```python
from build123d import *

# Parameters (mm, degrees)
SKETCH2_W           = 8.2
SKETCH2_H           = 8.3
SKETCH2_R           = 0.833443519
SKETCH2_R_2         = 0.823803164
BOSS_EXTRUDE1_DEPTH = 1.35
SKETCH3_W           = 1.2
SKETCH3_H           = 3.1
BOSS_EXTRUDE2_DEPTH = 0.25


with BuildPart() as part:
    # Sketch2 → Boss-Extrude1 (new body, symmetric)
    with BuildSketch(Plane.XY):
        Rectangle(SKETCH2_W, SKETCH2_H)
        with Locations((-2, -2.55)):
            Circle(SKETCH2_R, mode=Mode.SUBTRACT)
        with Locations((2, -2.55)):
            Circle(SKETCH2_R_2, mode=Mode.SUBTRACT)
    extrude(amount=BOSS_EXTRUDE1_DEPTH, both=True)

    # Sketch3 → Boss-Extrude2 (add, symmetric)
    with BuildSketch(Plane.XY):
        with Locations((0, -5.7)):
            Rectangle(SKETCH3_W, SKETCH3_H)
        with Locations((2.5, -5.7)):
            Rectangle(SKETCH3_W, SKETCH3_H)
        with Locations((-2.5, -5.7)):
            Rectangle(SKETCH3_W, SKETCH3_H)
    extrude(amount=BOSS_EXTRUDE2_DEPTH, both=True)


solid = part.part
```
Geometry check sheet. Reference: the model listing, model coordinates, mm. A direction names the side the tool comes from. Give positions to 0.01 mm unless a question says otherwise; leave off trailing zeros. Loops run counter-clockwise (first coordinate to the right, second up) from the corner with the lowest first, then second, coordinate; pieces in that order, holes last. Notation, with made-up numbers: (80.5, 68) - (100.5, 68) arc R21 ccw to (100.5, 91) - close; hole circle Ø3 at (34, 10). An arc over 180 degrees is marked (long way). Use CSV: the item, a comma, the result in double quotes. Start each with the question number.
Q1. Scan lines: probe 1 along Y at (x, z) = (-2, 0.6); probe 2 along Y at (x, z) = (2, 0.15); probe 3 along X at (y, z) = (-2.75, -0.6). Record each from-to range of solid material in increasing order. Write a range as from..to.
Q2. Section check A-A, the plane y = -2.55. Record the cut outline in (x, z), and give its area (3 significant figures).
Q3. Section check D-D, the plane x = -3.5. Record the cut outline in (y, z), and give its area (3 significant figures).
Q4. Section check B-B, the plane z = -0.1. Record the cut outline in (x, y), and give its area (3 significant figures).
Q5. Go/stop test with flat-tipped pins: pin 1 Ø0.6 at (y, z) = (-5.5, 0) entering from -X; pin 2 Ø1.3 at (x, y) = (2.5, -6.5) entering from -Z; pin 3 Ø1.3 at (x, y) = (-2.5, -5.5) entering from +Z; pin 4 Ø1.5 at (x, y) = (2, -2.55) entering from +Z. Record where each tip stops, or that it passes through.
Q6. Release check for a two-part mould opening along Y. For faces 4 (the face through (1.346, -3.051, -0.019)), 5 (the face through (4.1, 0, 0)), 6 (the face through (0, 4.15, 0)), 7 (the face through (-2.833, -2.513, -0.019)) record: +Y half, -Y half, draft (parallel to the pull), parting line (faces both ways), or undercut.
Q7. Section check C-C, the plane x = -1.75. Record the cut outline in (y, z).
Q8. Access from +Z, -Z, +X, -X, +Y, -Y to the whole of each face (thin tool, end or side, straight path). Record for faces 1 (the face through (-4.1, 0, 0)), 2 (the face through (-2.5, -5.7, -0.25)), 3 (the face through (0, -6, 0.25)).
Findings below:
1,probe 1,"y = -4.15..-3.38, -1.72..4.15"
1,probe 2,"y = -7.25..-3.37, -1.73..4.15"
1,probe 3,"x = -4.1..-2.81, -1.19..1.2, 2.8..4.1"
2,outline,"(-4.1, -1.35) - (-2.83, -1.35) - (-2.83, 1.35) - (-4.1, 1.35) - close; (-1.17, -1.35) - (1.18, -1.35) - (1.18, 1.35) - (-1.17, 1.35) - close; (2.82, -1.35) - (4.1, -1.35) - (4.1, 1.35) - (2.82, 1.35) - close"
2,area,"13.2 mm^2"
3,outline,"(-4.15, -1.35) - (4.15, -1.35) - (4.15, 1.35) - (-4.15, 1.35) - close"
3,area,"22.4 mm^2"
4,outline,"(-4.1, -4.15) - (-3.1, -4.15) - (-3.1, -7.25) - (-1.9, -7.25) - (-1.9, -4.15) - (-0.6, -4.15) - (-0.6, -7.25) - (0.6, -7.25) - (0.6, -4.15) - (1.9, -4.15) - (1.9, -7.25) - (3.1, -7.25) - (3.1, -4.15) - (4.1, -4.15) - (4.1, 4.15) - (-4.1, 4.15) - close; hole circle Ø1.67 at (-2, -2.55); hole circle Ø1.65 at (2, -2.55)"
4,area,"74.9 mm^2"
5,pin 1,"stops at x = -3.1"
5,pin 2,"stops at z = -0.25"
5,pin 3,"stops at z = 0.25"
5,pin 4,"passes through"
6,face 4,"undercut"
6,face 5,"draft"
6,face 6,"+Y half"
6,face 7,"undercut"
7,outline,"(-4.15, -1.35) - (-3.35, -1.35) - (-3.35, 1.35) - (-4.15, 1.35) - close; (-1.75, -1.35) - (4.15, -1.35) - (4.15, 1.35) - (-1.75, 1.35) - close"
8,face 1,"+Z, -Z, -X, +Y, -Y"
8,face 2,"-Z, +X, -X, -Y"
8,face 3,"+Z, +X, -X, -Y"
